Can you work these out from the model? Positions are in its coordinate system, mm. Round coordinates to 2 decimals unless told otherwise and drop trailing zeros. Answer in a Markdown table with one row per item. Add a question column.
(1) If I drill on probe 1 along Y at (x, z) = (-50, 17.5); probe 2 along Y at (x, z) = (48, 9.75), over which ranges is the centre line in solid material (lowest first)?
(2) Suppose I cut it at A-A, the plane x = -40. Count the separate pieces of the cut face and the enclosed holes in it, then the cut area to 3 significant figures.
(3) If we mould it in two halves opening along Y, with no side actions, what happens to faces 1 (the face through (-55.495, -44.758, 16.845)), 2 (the face through (-1, -14, 20)), 3 (the face through (37.69, 59.04, 9.86)), 4 (the face through (-1, 65, 10))? For each: released by +Y, released by -Y, zero draft, split by the parting line, or undercut.
from build123d import *

# Parameters (mm, degrees)
SKETCH1_W                                           = 130
SKETCH1_H                                           = 130
EXTRUDE1_DEPTH                                      = 20
M6_TAPPED_HOLE1_D                                   = 5
CBORE_FOR_M6_HEX_SOCKET_HEAD_CAP_SCREW1_D           = 6.6
CBORE_FOR_M6_HEX_SOCKET_HEAD_CAP_SCREW1_CBORE_D     = 11
CBORE_FOR_M6_HEX_SOCKET_HEAD_CAP_SCREW1_CBORE_DEPTH = 6.4


with BuildPart() as part:
    # Sketch1 → Extrude1 (new body)
    with BuildSketch(Plane.XY):
        Rectangle(SKETCH1_W, SKETCH1_H)
    extrude(amount=EXTRUDE1_DEPTH)

    # M6 Tapped Hole1 (through all)
    with Locations(Plane.XY.offset(20)):
        with Locations((-60, -60), (-40, -60), (-20, -60), (0, -60), (20, -60), (40, -60), (-40, -40), (-20, -40), (0, -40), (20, -40), (40, -40), (-40, -20), (-20, -20), (0, -20), (20, -20), (40, -20), (-40, 0), (-20, 0), (0, 0), (20, 0), (40, 0), (-40, 20), (-20, 20), (0, 20), (20, 20), (40, 20), (-40, 40), (-20, 40), (0, 40), (20, 40), (40, 40), (-40, 60), (-20, 60), (0, 60), (20, 60), (40, 60), (-60, -40), (-60, -20), (-60, 0), (-60, 20), (-60, 40), (-60, 60), (60, -60), (60, -40), (60, -20), (60, 0), (60, 20), (60, 40), (60, 60)):
            Hole(M6_TAPPED_HOLE1_D / 2)

    # CBORE for M6 Hex Socket Head Cap Screw1 (through all)
    with Locations(Plane.XY.offset(20)):
        with Locations((-50, 45), (50, 45), (50, -45), (-50, -45), (0, 0)):
            CounterBoreHole(CBORE_FOR_M6_HEX_SOCKET_HEAD_CAP_SCREW1_D / 2, CBORE_FOR_M6_HEX_SOCKET_HEAD_CAP_SCREW1_CBORE_D / 2, CBORE_FOR_M6_HEX_SOCKET_HEAD_CAP_SCREW1_CBORE_DEPTH)


solid = part.part
Calculated:
| question | item | result |
|---|---|---|
| 1 | probe 1 | -65 to -50.5, -39.5 to 39.5, 50.5 to 65 |
| 1 | probe 2 | -65 to -47.62, -42.38 to 42.38, 47.62 to 65 |
| 2 | separate pieces | 8 |
| 2 | enclosed holes | 0 |
| 2 | area | 1,900 mm² |
| 3 | face 1 | undercut |
| 3 | face 2 | zero draft |
| 3 | face 3 | undercut |
| 3 | face 4 | released by +Y |
